Autodesk Inventor part; units mm, degrees
ref_plane "YZ Plane" through (0, 0, 0) normal (1, 0, 0) x (0, 1, 0)
ref_plane "XZ Plane" through (0, 0, 0) normal (0, 1, 0) x (-1, 0, 0)
ref_plane "XY Plane" through (0, 0, 0) normal (0, 0, 1) x (1, 0, 0)
sketch "Sketch1" plane through (0, 0, 0) normal (0, 1, 0) x (-1, 0, 0)
  line L0 (-21.5, 21.5) -> (21.5, 21.5)
  line L1 (21.5, 21.5) -> (21.5, -21.5)
  line L2 (21.5, -21.5) -> (-21.5, -21.5)
  line L3 (-21.5, -21.5) -> (-21.5, 21.5)
  line L4 (-21.5, 21.5) -> (21.5, -21.5) construction
  line L5 (21.5, 21.5) -> (-21.5, -21.5) construction
  point P0 (0, 0)
  dimension "d0" = 43
  dimension "d1" = 43
extrude "Extrusion1" add sketch "Sketch1" along normal blind 21
sketch "Sketch2" plane through (0, 21, 0) normal (0, 1, 0) x (1, 0, 0)
  line L0 (21.5, 21.5) -> (-21.5, 21.5) construction
  line L1 (-21.5, 21.5) -> (-21.5, -21.5) construction
  line L2 (-21.5, -21.5) -> (21.5, -21.5) construction
  line L3 (21.5, -21.5) -> (21.5, 21.5) construction
  line L4 (21.5, -21.5) -> (-21.5, 21.5) construction
  line L5 (21.5, 21.5) -> (-21.5, -21.5) construction
  circle A0 centre (0, 0) radius 11
  dimension "d4" = 22
extrude "Extrusion2" add sketch "Sketch2" along normal blind 2
sketch "Sketch3" plane through (0, 23, 0) normal (0, 1, 0) x (1, 0, 0)
  circle A0 centre (0, 0) radius 11 construction
  circle A1 centre (0, 0) radius 11 construction
  circle A2 centre (0, 0) radius 2.5
  dimension "d7" = 5
extrude "Extrusion3" add sketch "Sketch3" along normal blind 18
sketch "Sketch4" plane through (0, 41, 0) normal (0, 1, 0) x (1, 0, 0)
  circle A0 centre (0, 0) radius 2.5
  line L0 (1.7854, 1.75) -> (1.7854, -1.75)
  dimension "d11" = 3.5
extrude "Extrusion4" cut sketch "Sketch4" against normal blind 16.75 contours A0 L0 picked at (1.8866, -0.4578)
chamfer "Chamfer1" distance 4.0426 angle 45 4 edges at (-21.5, 10.5, 21.5) (21.5, 10.5, 21.5) (21.5, 10.5, -21.5) (-21.5, 10.5, -21.5)
sketch "Sketch5" plane through (0, 21, 0) normal (0, 1, 0) x (1, 0, 0)
  line L0 (-21.5, 17.4574) -> (-17.4574, 21.5) construction
  line L1 (-21.5, 17.4574) -> (-21.5, -17.4574) construction
  line L2 (-17.4574, -21.5) -> (-21.5, -17.4574) construction
  line L3 (-17.4574, -21.5) -> (17.4574, -21.5) construction
  line L4 (21.5, -17.4574) -> (17.4574, -21.5) construction
  line L5 (21.5, -17.4574) -> (21.5, 17.4574) construction
  line L6 (17.4574, 21.5) -> (21.5, 17.4574) construction
  line L7 (17.4574, 21.5) -> (-17.4574, 21.5) construction
  circle A0 centre (0, 0) radius 11 construction
  line L8 (15.5, -15.5) -> (-15.5, -15.5) construction
  line L9 (-15.5, -15.5) -> (-15.5, 15.5) construction
  line L10 (-15.5, 15.5) -> (15.5, 15.5) construction
  line L11 (15.5, 15.5) -> (15.5, -15.5) construction
  circle A1 centre (0, 0) radius 2.5 construction
  line L12 (15.5, -15.5) -> (-15.5, 15.5) construction
  line L13 (-15.5, -15.5) -> (15.5, 15.5) construction
  dimension "d17" = 31
  dimension "d18" = 31
hole "Hole1" at (-15.5, 21, 15.5) at (-15.5, 21, -15.5) at (15.5, 21, -15.5) at (15.5, 21, 15.5) direction (0, -1, 0) diameter 2.459 depth 3.5
properties part number "PancakeStepper" material "Steel, Carbon"
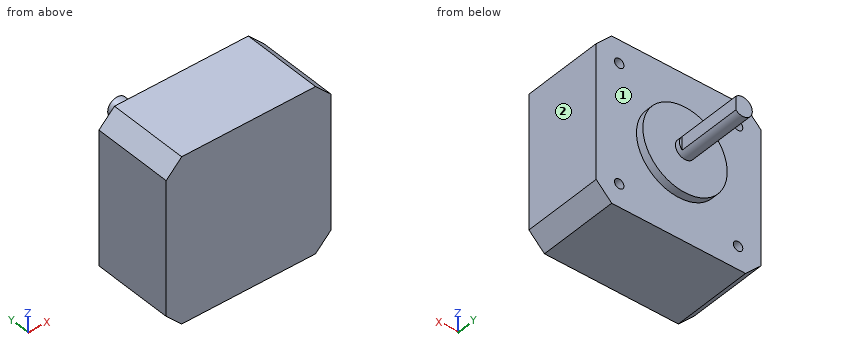
Check sheet for the modelled part. Datum: model origin and axes. Units: mm. Face numbers are marked on the shaded views. A direction names the side the tool comes from. Round coordinates to 2 decimals unless told otherwise and drop trailing zeros. Loops run counter-clockwise (first coordinate to the right, second up) from the corner with the lowest first, then second, coordinate; pieces in that order, holes last. Notation, with made-up numbers: (76.5, -32) - (128.5, -32) arc R12 ccw to (128.5, -14) - close; hole circle Ø7 at (-12.75, 51). An arc over 180 degrees is marked (long way). Answer as CSV lines item,"result". Start each with the question number.
Item 1: Set-up check for the marked faces 1 and 2: record each of +Z, -Z, +X, -X, +Y, -Y from which the full face is reachable in a straight line by a thin tool's end or side.
Item 2: Depth check by flat-ended pin: P1, Ø1.5, axis at x = 15.5, z = 15.5, coming from the +Y side; P2, Ø4, axis at y = 36, z = 0.5, coming from the +X side; P3, Ø6, axis at x = 2.5, z = 9.5, coming from the +Y side. Enter the tip coordinate at first touch or a pass-through.
Item 3: Section check A-A (y = 19). Record the boundary of the cut face in (x, z).
Item 4: Section check C-C (x = -5.5). Record the boundary of the cut face in (y, z), and give its area (3 significant figures).
Item 5: Section check D-D (y = 6). Record the boundary of the cut face in (x, z), and give its area (3 significant figures).
Item 6: Section check B-B (z = -15.5). Record the boundary of the cut face in (x, y).
Item 7: Scan lines: line 1 (Z direction, x = 15.5, y = 19.65); line 2 (Z direction, x = 15, y = 20). Record each from-to range of solid material in increasing order. Write a range as [from, to].
Report:
1,face 1,"+Y"
1,face 2,"+Z, -Z, +X, +Y, -Y"
2,P1,"stops at y = 17.5"
2,P2,"stops at x = 1.79"
2,P3,"stops at y = 23"
3,outline,"(-21.5, -17.46) - (-17.46, -21.5) - (17.46, -21.5) - (21.5, -17.46) - (21.5, 17.46) - (17.46, 21.5) - (-17.46, 21.5) - (-21.5, 17.46) - close; hole circle Ø2.46 at (-15.5, -15.5); hole circle Ø2.46 at (-15.5, 15.5); hole circle Ø2.46 at (15.5, -15.5); hole circle Ø2.46 at (15.5, 15.5)"
4,outline,"(0, -21.5) - (21, -21.5) - (21, -9.53) - (23, -9.53) - (23, 9.53) - (21, 9.53) - (21, 21.5) - (0, 21.5) - close"
4,area,"941 mm2"
5,outline,"(-21.5, -17.46) - (-17.46, -21.5) - (17.46, -21.5) - (21.5, -17.46) - (21.5, 17.46) - (17.46, 21.5) - (-17.46, 21.5) - (-21.5, 17.46) - close"
5,area,"1,820 mm2"
6,outline,"(-21.5, 0) - (21.5, 0) - (21.5, 21) - (16.73, 21) - (16.73, 17.5) - (14.27, 17.5) - (14.27, 21) - (-14.27, 21) - (-14.27, 17.5) - (-16.73, 17.5) - (-16.73, 21) - (-21.5, 21) - close"
7,line 1,"z = [-21.5, -16.73], [-14.27, 14.27], [16.73, 21.5]"
7,line 2,"z = [-21.5, -16.62], [-14.38, 14.38], [16.62, 21.5]"
